from build123d import *

# Parameters (mm, degrees)
SKETCH_1_W          = 43
SKETCH_1_H          = 43
EXTRUDE_1_DEPTH     = 1.5
SKETCH_2_R          = 1.75
CUT_EXTRUDE_1_DEPTH = 1.5
SKETCH_3_W          = 23
SKETCH_3_H          = 16
EXTRUDE_2_DEPTH     = 26


with BuildPart() as part:
    # 草图1 → 凸台-拉伸1 (new body)
    with BuildSketch(Plane(origin=(0, 0, 0), x_dir=(1, 0, 0), z_dir=(0, 1, 0))):
        Rectangle(SKETCH_1_W, SKETCH_1_H)
    extrude(amount=EXTRUDE_1_DEPTH)

    # 草图2 → 切除-拉伸1 (cut)
    with BuildSketch(Plane(origin=(0, 1.5, 0), x_dir=(1, 0, 0), z_dir=(0, 1, 0))):
        with Locations(Location((-18.5, 18.5, 0), (0, 0, 270))):
            Circle(SKETCH_2_R)
        with Locations(Location((18.5, 18.5, 0), (0, 0, 90))):
            Circle(SKETCH_2_R)
        with Locations(Location((-18.5, -18.5, 0), (0, 0, 90))):
            Circle(SKETCH_2_R)
        with Locations(Location((18.5, -18.5, 0), (0, 0, 270))):
            Circle(SKETCH_2_R)
    extrude(amount=-CUT_EXTRUDE_1_DEPTH, mode=Mode.SUBTRACT)

    # 草图3 → 凸台-拉伸2 (add)
    with BuildSketch(Plane(origin=(0, 1.5, 0), x_dir=(1, 0, 0), z_dir=(0, 1, 0))):
        with Locations((0, 13.5)):
            Rectangle(SKETCH_3_W, SKETCH_3_H)
    extrude(amount=EXTRUDE_2_DEPTH)


solid = part.part
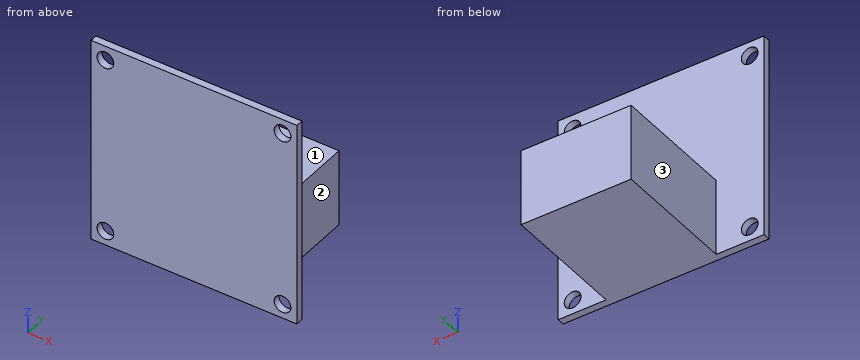
Work out the finished part from the listing and answer in its coordinate system (mm). Face numbers are marked on the shaded views. A direction names the side the tool comes from. Give positions to 0.01 mm unless a question says otherwise; leave off trailing zeros. Loops run counter-clockwise (first coordinate to the right, second up) from the corner with the lowest first, then second, coordinate; pieces in that order, holes last. Notation, with made-up numbers: (-18, -30.75) - (-1, -30.75) arc R32 cw to (-1, 2.25) - close; hole circle Ø6 at (85, 61.5). An arc over 180 degrees is marked (long way). Answer in a Markdown table with one row per item. Add a question column.
Q1. The part is cut by section A-A (z = 18.5). Determine the outline of the cut face in (x, y).
Q2. The part is cut by section D-D (z = -18.5). Determine the outline of the cut face in (x, y).
Q3. A tool of negligible diameter and unlimited length cuts with its end or side. For the marked faces 1, 2 and 3, from which of +Z, -Z, +X, -X, +Y, -Y can it reach the whole face along a straight path? Write none if from no direction.
Q4. The part is cut by section C-C (x = -4.5). Determine the outline of the cut face in (y, z).
Q5. Each of these flat-tipped pins is pushed along its axis until it touches: P1, Ø11.5, axis at x = 2.5, y = 17, coming from the +Z side; P2, Ø6, axis at x = -5, z = 15.5, coming from the +Y side; P3, Ø5, axis at x = 9.5, z = 10, coming from the -Y side; P4, Ø13, axis at y = 10, z = -14.5, coming from the -X side. Where does it stop, or does it pass through?
Q6. Consider line 1 along X through (y, z) = (0.3, -18.5); line 2 along Z through (x, y) = (-5.5, 4.25); line 3 along Y through (x, z) = (-18, -12). Determine where each line is inside the solid, lowest interval first.
Q7. The part is cut by section B-B (x = -18.5). Determine the outline of the cut face in (y, z).
Solution:
| question | item | result |
|---|---|---|
| 1 | outline | (-21.5, 0) - (-20.25, 0) - (-20.25, 1.5) - (-21.5, 1.5) - close; (-16.75, 0) - (16.75, 0) - (16.75, 1.5) - (-16.75, 1.5) - close; (20.25, 0) - (21.5, 0) - (21.5, 1.5) - (20.25, 1.5) - close |
| 2 | outline | (-21.5, 0) - (-20.25, 0) - (-20.25, 1.5) - (-21.5, 1.5) - close; (-16.75, 0) - (16.75, 0) - (16.75, 1.5) - (11.5, 1.5) - (11.5, 27.5) - (-11.5, 27.5) - (-11.5, 1.5) - (-16.75, 1.5) - close; (20.25, 0) - (21.5, 0) - (21.5, 1.5) - (20.25, 1.5) - close |
| 3 | face 1 | +Z, +X, -X, +Y |
| 3 | face 2 | +Z, -Z, +X, +Y |
| 3 | face 3 | +Z, -Z, -X, +Y |
| 4 | outline | (0, -21.5) - (27.5, -21.5) - (27.5, -5.5) - (1.5, -5.5) - (1.5, 21.5) - (0, 21.5) - close |
| 5 | P1 | stops at z = -5.5 |
| 5 | P2 | stops at y = 1.5 |
| 5 | P3 | stops at y = 0 |
| 5 | P4 | stops at x = -11.5 |
| 6 | line 1 | x = -21.5 to -20.25, -16.75 to 16.75, 20.25 to 21.5 |
| 6 | line 2 | z = -21.5 to -5.5 |
| 6 | line 3 | y = 0 to 1.5 |
| 7 | outline | (0, -21.5) - (1.5, -21.5) - (1.5, -20.25) - (0, -20.25) - close; (0, -16.75) - (1.5, -16.75) - (1.5, 16.75) - (0, 16.75) - close; (0, 20.25) - (1.5, 20.25) - (1.5, 21.5) - (0, 21.5) - close |
